Autodesk Inventor part; units mm, degrees
ref_plane "YZ Plane" through (0, 0, 0) normal (1, 0, 0) x (0, 1, 0)
ref_plane "XZ Plane" through (0, 0, 0) normal (0, 1, 0) x (-1, 0, 0)
ref_plane "XY Plane" through (0, 0, 0) normal (0, 0, 1) x (1, 0, 0)
sketch "Sketch1" plane through (0, 0, 0) normal (0, 0, 1) x (1, 0, 0)
  line L0 (0, 0) -> (-80, 0)
  line L1 (-80, 2) -> (0, 2)
  line L2 (0, 2) -> (0, 0)
  line L3 (-80, 2) -> (-84.2329, 2)
  line L4 (-133.3122, -28) -> (-131.553, -28)
  spline S0 degree 2 poles (-80, 0) (-102.6249, 1.8185) (-131.553, -28) knots 0 0 0 1 1 1
  spline S1 degree 2 poles (-80, 2) (-102.2926, 3.4342) (-135, -26) knots 0 0 0 1 1 1
  spline S2 degree 2 poles (-135, -26) (-137.4492, -28.2041) (-131.553, -28) knots 0 0 0 1 1 1
  line L5 (0, 1.35) -> (0, 1)
  line L6 (0, 0.65) -> (0, 1)
  point P0 (-99.9996, -4.0002)
  point P1 (-100, -1)
  point P2 (-100, -2)
  dimension "d1" = 2
extrude "Extrusion1" add sketch "Sketch1" along normal blind 1.2 contours L0 S0 L4 S2 S1 L3 L1 L2
sketch "Sketch2" plane through (0, 0, 0) normal (1, 0, 0) x (0, 0, -1)
  line L0 (-1.2, 0) -> (-1.2, 2)
  line L1 (0, 0) -> (0, 2)
  line L2 (0, 2) -> (-1.2, 2)
  line L3 (0.4, 0.85) -> (-1.6, 0.85)
  line L4 (-1.6, 0.85) -> (-1.6, 1.35)
  line L5 (-1.6, 1.35) -> (0.4, 1.35)
  line L6 (0.4, 1.35) -> (0.4, 0.85)
  line L7 (0.4, 0.85) -> (-1.6, 1.35) construction
  line L8 (-1.6, 0.85) -> (0.4, 1.35) construction
  point P0 (-0.6, 1.1)
  dimension "d12" = 2
  dimension "d13" = 0.5
extrude "Extrusion2" add sketch "Sketch2" along normal blind 2.5 contours L3 L4 L5 L0 | L0 L5 L1 L3 | L1 L5 L6 L3
sketch "Sketch3" plane through (0, 1.35, 0) normal (0, 1, 0) x (1, 0, 0)
  line L0 (0, 0) -> (0, -1.2)
  line L1 (0, 0.4) -> (2.5, 0.4)
  point P0 (1.25, -0.6)
hole "Hole1" at (1.25, 1.35, 0.6) direction (0, -1, 0) diameter 1.25 depth 0.7
fillet "Fillet1" radius 0.3 4 edges at (0, 1.675, 1.2) (0, 1.675, 0) (0, 0.425, 1.2) (0, 0.425, 0)
properties part number "brat bun ochelari" material "Iron, Cast"
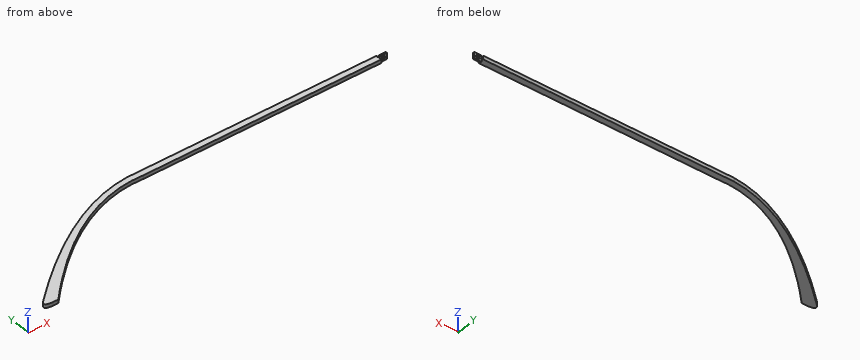
Input: part model. Units: mm. Frame: model coordinates. Give positions to 0.01 mm unless a question says otherwise; leave off trailing zeros. Write each loop counter-clockwise with the first axis right and the second up, starting at its lowest first coordinate (ties: lowest second). Pieces come first, ordered by that corner, then holes.
Q1. Material intervals for probe 1 along Z at (x, y) = (1.25, 1.15) (3 decimals); probe 2 along Y at (x, z) = (-29.5, 0.05); probe 3 along Z at (x, y) = (-107.5, -7), sorted ascending.
Q2. Section A-A, the plane x = -77.5. Output: boundary loops of the cut face in (y, z).
Q3. First-contact query: P1, Ø1, axis at y = -23, z = 1, coming from the -X side. Flat tip, straight axial feed; report the tip coordinate or a pass-through.
Filled in:
1. probe 1: z = -0.4 to -0.025, 1.225 to 1.6
1. probe 2: y = 0 to 2
1. probe 3: z = 0 to 1.2
2. outline: (0, 0) - (2, 0) - (2, 1.2) - (0, 1.2) - close
3. P1: stops at x = -132.18
